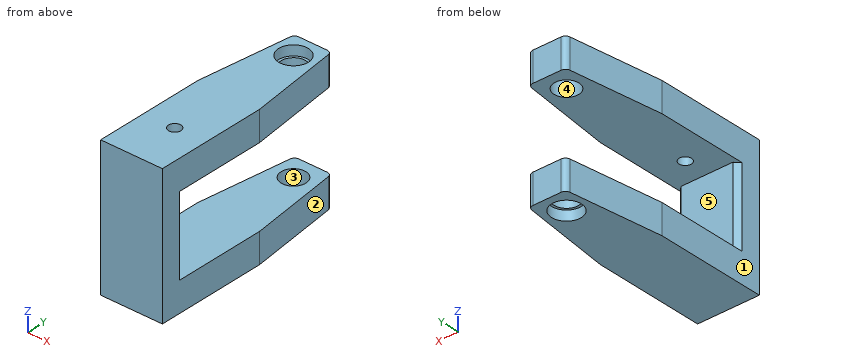
from build123d import *

# Parameters (mm, degrees)
BOSS_EXTRUDE2_DEPTH   = 28
SKETCH16_W            = 32
SKETCH16_H            = 74
CUT_EXTRUDE3_DEPTH    = 26
M6_TAPPED_HOLE1_D     = 5
M6_TAPPED_HOLE1_DEPTH = 27
M6_TAPPED_HOLE1_TIP   = 1.502151548
CHAMFER1_SIZE         = 2
FILLET1_R             = 2


with BuildPart() as part:
    # Sketch15 → Boss-Extrude2 (new body, symmetric)
    with BuildSketch(Plane.XY):
        Polygon((-12.5, 0), (12.5, 0), (12.5, 45), (7.5, 84), (-7.5, 84), (-12.5, 45), align=None)
    extrude(amount=BOSS_EXTRUDE2_DEPTH, both=True)

    # Sketch16 → Cut-Extrude3 (cut, through all)
    with BuildSketch(Plane(origin=(12.5, 0, 0), x_dir=(0, 0, -1), z_dir=(1, 0, 0))):
        with Locations((0, 47)):
            Rectangle(SKETCH16_W, SKETCH16_H)
    extrude(amount=-CUT_EXTRUDE3_DEPTH, mode=Mode.SUBTRACT)

    # Sketch18 → CBORE for M4 Hex Socket Head Cap Screw1 (revolve, cut)
    with BuildSketch(Plane(origin=(0, 75, 28), x_dir=(0, -1, 0), z_dir=(1, 0, 0))):
        Polygon((0, 0), (0, 23.004303095), (5, 20), (5, 4), (6, 4), (6, 0), align=None)
    cbore_for_m4_hex_socket_head_cap_screw1 = revolve(axis=Axis((0, 75, 34.35), (0, 0, -1)), mode=Mode.SUBTRACT)

    # Mirror1: CBORE for M4 Hex Socket Head Cap Screw1 across plane
    add(cbore_for_m4_hex_socket_head_cap_screw1.mirror(Plane.XY), mode=Mode.SUBTRACT)

    # M6 Tapped Hole1
    with Locations(Plane.XY.offset(28)):
        with Locations((0, 20)):
            Hole(M6_TAPPED_HOLE1_D / 2, depth=M6_TAPPED_HOLE1_DEPTH)
            with Locations((0, 0, -(M6_TAPPED_HOLE1_DEPTH + M6_TAPPED_HOLE1_TIP / 2))):  # 118° drill point
                Cone(0, M6_TAPPED_HOLE1_D / 2, M6_TAPPED_HOLE1_TIP, mode=Mode.SUBTRACT)

    # Chamfer1
    chamfer1_edges = [part.edges().sort_by_distance(p)[0] for p in [
        (12.5, 10, 0),
        (-12.5, 10, 0),
    ]]
    chamfer(chamfer1_edges, length=CHAMFER1_SIZE)

    # Fillet1
    fillet1_edges = [part.edges().sort_by_distance(p)[0] for p in [
        (-7.5, 84, 22),
        (7.5, 84, 22),
        (-7.5, 84, -22),
        (7.5, 84, -22),
    ]]
    fillet(fillet1_edges, radius=FILLET1_R)


solid = part.part
The listing builds one solid part. Answer for the finished solid, in the listing's coordinates (mm). Face numbers are marked on the shaded views. A direction names the side the tool comes from. Round coordinates to 2 decimals unless told otherwise and drop trailing zeros. Write each loop counter-clockwise with the first axis right and the second up, starting at its lowest first coordinate (ties: lowest second). Pieces come first, ordered by that corner, then holes. Notation, with made-up numbers: M 13,19.5 L 50,19.5 A25 ccw 50,38.5 Z; hole C 14.25,56.25 d4. An arc over 180 degrees is marked long. Write each question's results on one line, items separated by ' | '. Start each with the question number.
Item 1: Straight lines are drawn through the part: probe 1 along Y at (x, z) = (0.25, 25); probe 2 along Y at (x, z) = (0, 22.5); probe 3 along Z at (x, y) = (1, 58.5). For each, find the intervals that lie inside material, in ascending order.
Item 2: Find section B-B on x = 0. Write down the section's boundary in (y, z).
Item 3: Find section C-C on z = 18. Write down the section's boundary in (x, y).
Item 4: Find section D-D on y = 56. Write down the section's boundary in (x, z), and give its area (3 significant figures).
Item 5: Which of the six approach directions +Z, -Z, +X, -X, +Y, -Y give full straight-line access (tool end or side, diameter ignored) to the marked faces 4 and 5?
Item 6: Find section A-A on y = 20. Write down the section's boundary in (x, z), and give its area (3 significant figures).
Item 7: The mould has two halves that part along Y. Classify the marked faces 1, 2 and 3: +Y half, -Y half, draft (parallel to the pull), parting line (faces both ways), or undercut.
Item 8: Given pin 1 Ø11.5 at (x, y) = (0, 75) entering from -Z; pin 2 Ø1.5 at (x, z) = (1.5, -4) entering from +Y, each flat-ended and moving along its own axis, determine where each tip first touches the part or whether it passes through.
Answer block:
1) probe 1: y = 0 to 17.51, 22.49 to 69.01, 80.99 to 84 | probe 2: y = 0 to 17.5, 22.5 to 70, 80 to 84 | probe 3: z = -28 to -16, 16 to 28
2) outline: M 0,-28 L 69,-28 L 69,-24 L 70,-24 L 70,-16 L 10,-16 L 10,16 L 17.5,16 L 17.5,28 L 0,28 Z; M 22.5,16 L 70,16 L 70,24 L 69,24 L 69,28 L 22.5,28 Z; M 80,-24 L 81,-24 L 81,-28 L 84,-28 L 84,-16 L 80,-16 Z; M 80,16 L 84,16 L 84,28 L 81,28 L 81,24 L 80,24 Z
3) outline: M -12.5,0 L 12.5,0 L 12.5,45 L 7.72,82.25 A2 ccw 5.74,84 L -5.74,84 A2 ccw -7.72,82.25 L -12.5,45 Z; hole C 0,75 d10; hole C 0,20 d5
4) outline: M -11.09,-28 L 11.09,-28 L 11.09,-16 L -11.09,-16 Z; M -11.09,16 L 11.09,16 L 11.09,28 L -11.09,28 Z | area: 532 mm²
5) face 4: +Z, -Z | face 5: +X, -X, +Y
6) outline: M -12.5,-28 L 12.5,-28 L 12.5,-16 L -12.5,-16 Z; M -12.5,16 L -2.5,16 L -2.5,28 L -12.5,28 Z; M 2.5,16 L 12.5,16 L 12.5,28 L 2.5,28 Z | area: 540 mm²
7) face 1: draft | face 2: +Y half | face 3: undercut
8) pin 1: stops at z = -24 | pin 2: stops at y = 10
